Check sheet for the modelled part. Datum: model origin and axes. Units: mm. Face numbers are marked on the shaded views. Coordinates: 2 decimals unless noted, no trailing zeros. Write each loop counter-clockwise with the first axis right and the second up, starting at its lowest first coordinate (ties: lowest second). Pieces come first, ordered by that corner, then holes. Notation, with made-up numbers: (87.25, 45.5) - (142.25, 45.5) arc R22 ccw to (142.25, 69.5) - close; hole circle Ø10 at (47.25, 22). An arc over 180 degrees is marked (long way). Use one line per item in the form item = value. Start each with the question number.
1. Cross-section at D-D on x = 8. Record the boundary of the cut face in (y, z), then the cut area to 3 significant figures.
2. Go/stop test with flat-tipped pins: pin 1 Ø7 at (x, y) = (-56.6, -90.4) entering from +Z; pin 2 Ø5.5 at (x, z) = (52, 19.5) entering from -Y; pin 3 Ø7.5 at (y, z) = (-60, 14) entering from -X. Record where each tip stops, or that it passes through.
3. Cross-section at C-C on z = 7.5. Give the number of separate pieces and of enclosed holes in the cut face, then the cut area to 3 significant figures.
4. Draft check along X on the marked faces 1 and 2. Enter one of: +X half, -X half, draft (parallel to the pull), parting line (faces both ways), or undercut.
5. Cross-section at A-A on y = 40. Record the boundary of the cut face in (x, z), then the cut area to 3 significant figures.
6. Scan lines: line 1 along Y through (x, z) = (-30, 3.5); line 2 along X through (y, z) = (-39.5, 3); line 3 along Y through (x, z) = (40, 3.5). Record each from-to range of solid material in increasing order.
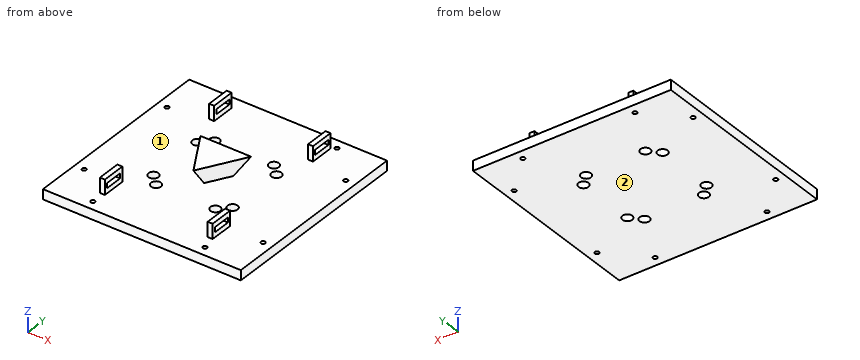
```python
from build123d import *

# Parameters (mm, degrees)
SKETCH1_W               = 200
SKETCH1_H               = 200
BOSS_EXTRUDE1_DEPTH     = 10
SKETCH2_R               = 5
SKETCH2_R_2             = 2.15
CUT_EXTRUDE1_DEPTH      = 142.774468788
BOSS_EXTRUDE2_DEPTH     = 20
DRAFT3_ANGLE            = -20
SKETCH6_W               = 5
SKETCH6_H               = 23.898224132
BOSS_EXTRUDE3_DEPTH     = 15
CUT_EXTRUDE3_DEPTH      = 185.814095783
CUT_EXTRUDE3_DEPTH_BACK = 185.814095783
SKETCH7_W               = 5
SKETCH7_H               = 18


with BuildPart() as part:
    # Sketch1 → Boss-Extrude1 (new body)
    with BuildSketch(Plane.XY):
        Rectangle(SKETCH1_W, SKETCH1_H)
    extrude(amount=BOSS_EXTRUDE1_DEPTH)

    # Sketch2 → Cut-Extrude1 (cut, through all)
    with BuildSketch(Plane.XY.offset(10)):
        with Locations((-40, 30)):
            Circle(SKETCH2_R)
        with Locations((40, 30)):
            Circle(SKETCH2_R)
        with Locations((40, -30)):
            Circle(SKETCH2_R)
        with Locations((-40, -30)):
            Circle(SKETCH2_R)
        with Locations((-30, 40)):
            Circle(SKETCH2_R)
        with Locations((30, 40)):
            Circle(SKETCH2_R)
        with Locations((30, -40)):
            Circle(SKETCH2_R)
        with Locations((-30, -40)):
            Circle(SKETCH2_R)
        with Locations((-56.6, 90.4)):
            Circle(SKETCH2_R_2)
        with Locations((-90.4, 56.6)):
            Circle(SKETCH2_R_2)
        with Locations((-90.4, -56.6)):
            Circle(SKETCH2_R_2)
        with Locations((-56.6, -90.4)):
            Circle(SKETCH2_R_2)
        with Locations((56.6, -90.4)):
            Circle(SKETCH2_R_2)
        with Locations((90.4, -56.6)):
            Circle(SKETCH2_R_2)
        with Locations((90.4, 56.6)):
            Circle(SKETCH2_R_2)
        with Locations((56.6, 90.4)):
            Circle(SKETCH2_R_2)
    extrude(amount=-CUT_EXTRUDE1_DEPTH, mode=Mode.SUBTRACT)

    # Sketch4 → Boss-Extrude2 (add)
    with BuildSketch(Plane.XY.offset(10)):
        Polygon((0, -15), (12.990381057, 7.5), (-12.990381057, 7.5), align=None)
    extrude(amount=BOSS_EXTRUDE2_DEPTH)

    # Draft3
    draft3_faces = [part.faces().sort_by_distance(p)[0] for p in [
        (0, 7.5, 20),
        (-6.495190528, -3.75, 20),
        (6.495190528, -3.75, 20),
    ]]
    draft(draft3_faces, Plane.XY.offset(10), DRAFT3_ANGLE)

    # Sketch6 → Boss-Extrude3 (add)
    with BuildSketch(Plane.XY.offset(10)):
        with Locations((50, 75)):
            Rectangle(SKETCH6_W, SKETCH6_H)
        with Locations((-50, 75)):
            Rectangle(SKETCH6_W, SKETCH6_H)
        with Locations((-57.033087887, -65)):
            Rectangle(SKETCH6_W, SKETCH6_H)
        with Locations((51.971023082, -65)):
            Rectangle(SKETCH6_W, SKETCH6_H)
    extrude(amount=BOSS_EXTRUDE3_DEPTH)

    # Sketch7 → Cut-Extrude3 (cut, two sides: drawn at the far end of the back side and taken through both)
    with BuildSketch(Plane(origin=(52.5, 0, 0), x_dir=(0, 0, -1), z_dir=(1, 0, 0)).offset(-CUT_EXTRUDE3_DEPTH_BACK)):
        with Locations((-17.5, 75)):
            Rectangle(SKETCH7_W, SKETCH7_H)
        with Locations((-17.5, -65)):
            Rectangle(SKETCH7_W, SKETCH7_H)
    extrude(amount=CUT_EXTRUDE3_DEPTH + CUT_EXTRUDE3_DEPTH_BACK, mode=Mode.SUBTRACT)


solid = part.part
```
Final values:
q1.outline = (-100, 0) - (100, 0) - (100, 10) - (7.5, 10) - (14.78, 30) - (-15.7, 30) - (-1.14, 10) - (-100, 10) - close
q1.area = 2,390 mm²
q2.pin_1 = 10
q2.pin_2 = -76.95
q2.pin_3 = -59.53
q3.separate_pieces = 1
q3.enclosed_holes = 16
q3.area = 39,300 mm²
q4.face_1 = undercut
q4.face_2 = draft
q5.outline = (-100, 0) - (-35, 0) - (-35, 10) - (-100, 10) - close; (-25, 0) - (25, 0) - (25, 10) - (-25, 10) - close; (35, 0) - (100, 0) - (100, 10) - (35, 10) - close
q5.area = 1,800 mm²
q6.line_1 = -100 to -45, -35 to 35, 45 to 100
q6.line_2 = -100 to -34.97, -25.03 to 25.03, 34.97 to 100
q6.line_3 = -100 to -35, -25 to 25, 35 to 100
